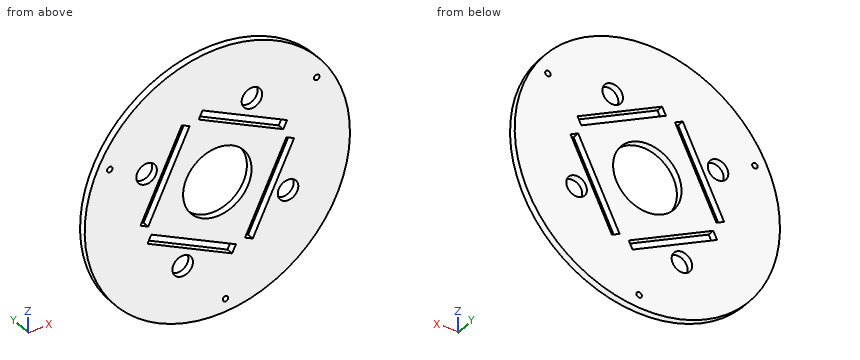
```python
from build123d import *

# Parameters (mm, degrees)
SKETCH_1_R               = 77.5
SKETCH_1_R_2             = 1.6
EXTRUDE_1_DEPTH          = 4
CUT_EXTRUDE_2_DEPTH      = 110.674518463
CUT_EXTRUDE_2_DEPTH_BACK = 110.674518463
SKETCH_3_R               = 20
CUT_EXTRUDE_3_DEPTH      = 110.674518463
CUT_EXTRUDE_3_DEPTH_BACK = 110.674518463
SKETCH_4_R               = 6


with BuildPart() as part:
    # 草图1 → 凸台-拉伸1 (new body)
    with BuildSketch(Plane(origin=(0, 0, 0), x_dir=(1, 0, 0), z_dir=(0, 1, 0))):
        with Locations(Location((0, 0, 0), (0, 0, 270))):
            Circle(SKETCH_1_R)
        with Locations(Location((4.784441198, 69.836302325, 0), (0, 0, 270))):
            Circle(SKETCH_1_R_2, mode=Mode.SUBTRACT)
        with Locations(Location((-62.872232519, -30.774703542, 0), (0, 0, 270))):
            Circle(SKETCH_1_R_2, mode=Mode.SUBTRACT)
        with Locations(Location((58.087791321, -39.061598783, 0), (0, 0, 270))):
            Circle(SKETCH_1_R_2, mode=Mode.SUBTRACT)
    extrude(amount=EXTRUDE_1_DEPTH)

    # 草图3 → 切除-拉伸2 (cut, two sides: drawn at the far end of the back side and taken through both)
    with BuildSketch(Plane(origin=(0, 4, 0), x_dir=(1, 0, 0), z_dir=(0, 1, 0)).offset(-CUT_EXTRUDE_2_DEPTH_BACK)):
        with Locations(Location((0, 0, 0), (0, 0, 270))):
            Circle(SKETCH_3_R)
    extrude(amount=CUT_EXTRUDE_2_DEPTH + CUT_EXTRUDE_2_DEPTH_BACK, mode=Mode.SUBTRACT)

    # 草图4 → 切除-拉伸3 (cut, two sides: drawn at the far end of the back side and taken through both)
    with BuildSketch(Plane.XZ.offset(-CUT_EXTRUDE_3_DEPTH_BACK)):
        with Locations(Location((-41.314039797, 20.194571008, 0), (0, 0, 270))):
            Circle(SKETCH_4_R)
        Polygon((-20.69437357, 40.719305585), (-44.874497782, -8.680305679), (-40.383624031, -10.87849879), (-16.203499819, 38.521112475), align=None)
        Polygon((-10.847694468, 40.35681714), (13.852111164, 28.266755034), (16.050304274, 32.757628786), (-8.649501358, 44.847690892), align=None)
        with Locations(Location((20.225375329, 41.287232906, 0), (0, 0, 270))):
            Circle(SKETCH_4_R)
        Polygon((13.852111164, 28.266755034), (38.551916796, 16.176692928), (40.750109907, 20.66756668), (16.050304274, 32.757628786), align=None)
        Polygon((20.698371001, -40.776916797), (44.878495213, 8.622694468), (40.387621462, 10.820887578), (16.20749725, -38.578723687), align=None)
        with Locations(Location((41.318037228, -20.252182219, 0), (0, 0, 270))):
            Circle(SKETCH_4_R)
        Polygon((-40.746112475, -20.725177891), (8.653498789, -44.905302103), (10.851691899, -40.414428352), (-38.547919365, -16.23430414), align=None)
        with Locations(Location((-20.221377898, -41.344844118, 0), (0, 0, 270))):
            Circle(SKETCH_4_R)
    extrude(amount=CUT_EXTRUDE_3_DEPTH + CUT_EXTRUDE_3_DEPTH_BACK, mode=Mode.SUBTRACT)


solid = part.part
```
The listing builds one solid part. Answer for the finished solid, in the listing's coordinates (mm). Coordinates: 2 decimals unless noted, no trailing zeros. Loops run counter-clockwise (first coordinate to the right, second up) from the corner with the lowest first, then second, coordinate; pieces in that order, holes last. Notation, with made-up numbers: (47, 22.25) -> (91, 22.25) arc R30 ccw to (91, 50.25) -> close; hole circle Ø8 at (85, -32). An arc over 180 degrees is marked (long way). Return JSON: item names as keys, results as strings. Group by question number.
(1) Given pin 1 Ø9.5 at (x, z) = (-20.22, -41.34) entering from +Y; pin 2 Ø1 at (y, z) = (1.5, 54.5) entering from -X; pin 3 Ø2 at (x, y) = (-4, 1) entering from -Z, each flat-ended and moving along its own axis, determine where each tip first touches the part or whether it passes through.
(2) Find the intervals of material crossed by probe 1 along Z at (x, y) = (28, 3.55); probe 2 along X at (y, z) = (1.1, 37); probe 3 along Z at (x, y) = (-22.5, 2.5), in increasing order. Write a range as from..to.
(3) A cutting plane is placed at C-C on y = 2. Count the separate pieces of the cut face and the enclosed holes in it, and give its area (3 significant figures).
(4) A cutting plane is placed at A-A on z = 0. Write down the section's boundary in (x, y).
(5) A cutting plane is placed at D-D on x = 0. Write down the section's boundary in (y, z), and give its area (3 significant figures).
(6) A cutting plane is placed at B-B on x = -28. Write down the section's boundary in (y, z).
The answers:
{
 "1": {"pin 1": "passes through", "pin 2": "stops at x = -55.59", "pin 3": "stops at z = -77.44"},
 "2": {"probe 1": "z = -72.27..-25.86, -14.49..21.34, 26.91..72.27", "probe 2": "x = -68.1..-22.51, -16.95..-3.99, 7.38..16.03, 24.42..68.1", "probe 3": "z = -74.16..-46.9, -35.79..-29.66, -24.09..25.66, 37.03..74.16"},
 "3": {"separate pieces": "1", "enclosed holes": "12", "area": "16,000 mm^2"},
 "4": {"outline": "(-77.5, 0) -> (-40.63, 0) -> (-40.63, 4) -> (-77.5, 4) -> close; (-35.06, 0) -> (-20, 0) -> (-20, 4) -> (-35.06, 4) -> close; (20, 0) -> (35.09, 0) -> (35.09, 4) -> (20, 4) -> close; (40.66, 0) -> (77.5, 0) -> (77.5, 4) -> (40.66, 4) -> close"},
 "5": {"outline": "(0, -77.5) -> (4, -77.5) -> (4, -40.67) -> (0, -40.67) -> close; (0, -35.1) -> (4, -35.1) -> (4, -20) -> (0, -20) -> close; (0, 20) -> (4, 20) -> (4, 35.05) -> (0, 35.05) -> close; (0, 40.61) -> (4, 40.61) -> (4, 77.5) -> (0, 77.5) -> close", "area": "415 mm^2"},
 "6": {"outline": "(0, -72.27) -> (4, -72.27) -> (4, -26.96) -> (0, -26.96) -> close; (0, -21.4) -> (4, -21.4) -> (4, 14.42) -> (0, 14.42) -> close; (0, 25.79) -> (4, 25.79) -> (4, 72.27) -> (0, 72.27) -> close"}
}
